from build123d import *

# Parameters (mm, degrees)
SKETCH3_R               = 8
BOSS_EXTRUDE1_DEPTH     = 31.578947368
CUT_EXTRUDE1_DEPTH      = 12.240009257
CUT_EXTRUDE1_DEPTH_BACK = 12.240009257
BOSS_EXTRUDE2_DEPTH     = 1.2
CUT_EXTRUDE2_DEPTH      = 1.6
SKETCH8_R               = 1.4
SKETCH8_R_2             = 1.6
CUT_EXTRUDE3_DEPTH      = 2.64160469
CUT_EXTRUDE3_DEPTH_BACK = 35.921940493
CUT_EXTRUDE4_DEPTH      = 35.921940493


with BuildPart() as part:
    # Sketch3 → Boss-Extrude1 (new body)
    with BuildSketch(Plane(origin=(-20.344467381, 196.178792599, 0), x_dir=(-0.994665758, -0.103150523, 0), z_dir=(0.103150523, -0.994665758, 0))):
        with Locations((-10.431405186, 0)):
            Circle(SKETCH3_R)
    extrude(amount=BOSS_EXTRUDE1_DEPTH)

    # Sketch4 → Cut-Extrude1 (cut, two sides)
    with BuildSketch(Plane(origin=(10.375761543, 1.076004901, 0), x_dir=(0.103150523, -0.994665758, 0), z_dir=(-0.994665758, -0.103150523, 0))) as cut_extrude1_sk:
        Polygon((-197.230869842, 0), (-189.230869842, 8), (-197.230869842, 8), align=None)
        Polygon((-173.651922474, 8), (-165.651922474, 8), (-165.651922474, 0), align=None)
    extrude(amount=CUT_EXTRUDE1_DEPTH, mode=Mode.SUBTRACT)
    extrude(cut_extrude1_sk.sketch, amount=-CUT_EXTRUDE1_DEPTH_BACK, mode=Mode.SUBTRACT)

    # Sketch5 → Boss-Extrude2 (add, symmetric)
    with BuildSketch(Plane(origin=(10.375761543, 1.076004901, 0), x_dir=(0.103150523, -0.994665758, 0), z_dir=(-0.994665758, -0.103150523, 0))):
        with BuildLine():
            Line((-165.651922474, -2.8), (-163.227051343, 1.4))
            ThreePointArc((-163.227051343, 1.4), (-165.286449135, 2.776045612), (-167.631821461, 1.979898987))
            Line((-167.631821461, 1.979898987), (-165.651922474, 0))
            Line((-165.651922474, 0), (-165.651922474, -2.8))
        make_face()
    extrude(amount=BOSS_EXTRUDE2_DEPTH, both=True)

    # Sketch7 → Cut-Extrude2 (cut, symmetric)
    with BuildSketch(Plane(origin=(10.375761543, 1.076004901, 0), x_dir=(0.103150523, -0.994665758, 0), z_dir=(-0.994665758, -0.103150523, 0))):
        with BuildLine():
            Line((-194.968128142, 2.2627417), (-197.230869842, 0))
            Line((-197.230869842, 0), (-197.230869842, -3.2))
            ThreePointArc((-197.230869842, -3.2), (-194.274455338, -1.224586984), (-194.968128142, 2.2627417))
        make_face()
    extrude(amount=CUT_EXTRUDE2_DEPTH, both=True, mode=Mode.SUBTRACT)

    # Sketch8 → Cut-Extrude3 (cut, two sides)
    with BuildSketch(Plane(origin=(-20.344467381, 196.178792599, 0), x_dir=(0.994665758, 0.103150523, 0), z_dir=(-0.103150523, 0.994665758, 0))) as cut_extrude3_sk:
        with Locations((10.431405186, -5.5)):
            Circle(SKETCH8_R)
        with Locations((6.831405186, 3)):
            Circle(SKETCH8_R_2)
        with Locations((14.031405186, 3)):
            Circle(SKETCH8_R_2)
    extrude(amount=CUT_EXTRUDE3_DEPTH, mode=Mode.SUBTRACT)
    extrude(cut_extrude3_sk.sketch, amount=-CUT_EXTRUDE3_DEPTH_BACK, mode=Mode.SUBTRACT)

    # Sketch9 → Cut-Extrude4 (cut, through all)
    with BuildSketch(Plane(origin=(-20.344467381, 196.178792599, 0), x_dir=(0.994665758, 0.103150523, 0), z_dir=(-0.103150523, 0.994665758, 0))):
        with BuildLine():
            Line((7.933405986, 7.6), (12.929404385, 7.6))
            ThreePointArc((12.929404385, 7.6), (10.431405186, 8), (7.933405986, 7.6))
        make_face()
        with BuildLine():
            Line((7.933405986, -7.6), (12.929404385, -7.6))
            ThreePointArc((12.929404385, -7.6), (10.431405186, -8), (7.933405986, -7.6))
        make_face()
    extrude(amount=-CUT_EXTRUDE4_DEPTH, mode=Mode.SUBTRACT)


solid = part.part
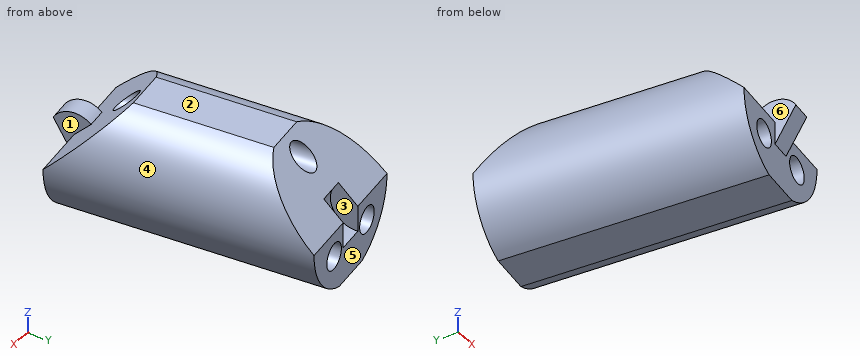
The listing builds one solid part. Answer for the finished solid, in the listing's coordinates (mm). Face numbers are marked on the shaded views. A direction names the side the tool comes from. Give positions to 0.01 mm unless a question says otherwise; leave off trailing zeros. Loops run counter-clockwise (first coordinate to the right, second up) from the corner with the lowest first, then second, coordinate; pieces in that order, holes last. Notation, with made-up numbers: (80, 29) - (97, 29) arc R18 cw to (97, 37) - close; hole circle Ø2 at (-16, 46). An arc over 180 degrees is marked (long way). Use one line per item in the form item = value.
1. Find the intervals of material crossed by line 1 along X through (y, z) = (188.5, -2.5); line 2 along X through (y, z) = (168.5, -3); line 3 along X through (y, z) = (174.5, 5), in increasing order. Write a range as [from, to].
Calculated:
line_1 = [-16.7, -14.21], [-11.15, -6.97], [-3.91, -1.42]
line_2 = [-14.44, -12.21], [-9, -4.98], [-1.76, 0.47]
line_3 = [-13.89, -8.92], [-6.29, -1.33]
2. Which of the six approach directions +Z, -Z, +X, -X, +Y, -Y give full straight-line access (tool end or side, diameter ignored) to the marked faces 1, 2 and 3?
Calculated:
face_1 = +Z, +X
face_2 = +Z, +X, -X, +Y, -Y
face_3 = +Y
3. Given pin 1 Ø1 at (x, y) = (-13, 188.5) entering from +Z; pin 2 Ø6 at (x, z) = (-6, -3) entering from +Y; pin 3 Ø4 at (x, z) = (-6.5, -0.5) entering from +Y, each flat-ended and moving along its own axis, determine where each tip first touches the part or whether it passes through.
Calculated:
pin_1 = 7.23
pin_2 = 197.98
pin_3 = 197.82
4. Section B-B on z = 0.75 is taken. Give the vertices of the cut face in (x, y).
Calculated:
outline = (-17.81, 195.69) - (-14.71, 165.77) - (-7.98, 166.47) - (-7.69, 163.68) - (-5.31, 163.93) - (-5.6, 166.71) - (1.13, 167.41) - (-1.97, 197.33) - (-8.3, 196.67) - (-8.06, 194.33) - (-11.24, 194) - (-11.48, 196.34) - close
5. Section C-C on y = 184 is taken. Count the separate pieces of the cut face and the enclosed holes in it, then the cut area to 3 significant figures.
Calculated:
separate_pieces = 1
enclosed_holes = 3
area = 177 mm^2
6. Section A-A on z = -1.75 is taken. Give the vertices of the cut face in (x, y), then the cut area to 3 significant figures.
Calculated:
outline = (-17.73, 196.45) - (-14.48, 165.04) - (-11.29, 165.37) - (-14.54, 196.78) - close; (-12.56, 196.99) - (-9.3, 165.58) - (-7.9, 165.72) - (-7.84, 165.12) - (-5.46, 165.37) - (-5.52, 165.97) - (-4.12, 166.11) - (-7.38, 197.52) - (-8.38, 197.42) - (-8.1, 194.76) - (-11.28, 194.42) - (-11.56, 197.09) - close; (-5.39, 197.73) - (-2.14, 166.32) - (1.05, 166.65) - (-2.2, 198.06) - close
area = 360 mm^2
7. The mould has two halves that part along X. Classify the marked faces 4, 5 and 6: pulls with the +X half, pulls with the -X half, needs draft (parallel to the pull), parting line crosses it, or undercut.
Calculated:
face_4 = pulls with the +X half
face_5 = pulls with the -X half
face_6 = undercut
